Here's how the part is built. I have some questions about the finished solid (model axes, mm). Coordinates: 2 decimals unless noted, no trailing zeros. Write each loop counter-clockwise with the first axis right and the second up, starting at its lowest first coordinate (ties: lowest second). Pieces come first, ordered by that corner, then holes. Notation, with made-up numbers: M 5,-10 L 62,-10 A28 cw 62,10 Z; hole C 34,30 d6. An arc over 180 degrees is marked long. Use one line per item in the form item = value. Start each with the question number.
1. I want a section at C-C, the plane x = 12. List the corners of the cut face in (y, z) for me, plus the area to 3 significant figures.
2. Please list where these lines run through material, in increasing order: line 1 along X through (y, z) = (0.3, 8); line 2 along X through (y, z) = (0.7, -5); line 3 along Z through (x, y) = (27, 0.65). Write a range as [from, to].
3. I want a section at A-A, the plane z = -3.5. List the corners of the cut face in (x, y) for me.
4. I want a section at B-B, the plane y = 0.2. List the corners of the cut face in (x, z) for me, plus the area to 3 significant figures.
from build123d import *

# Parameters (mm, degrees)
SKETCH1_W            = 240
SKETCH1_H            = 65
BOSS_EXTRUDE1_DEPTH  = 1
M4_CLEARANCE_SLOT1_D = 4.8
SKETCH4_R            = 17.5
CUT_EXTRUDE1_DEPTH   = 5


with BuildPart() as part:
    # Sketch1 → Boss-Extrude1 (new body)
    with BuildSketch(Plane(origin=(0, 0, 0), x_dir=(1, 0, 0), z_dir=(0, 1, 0))):
        with Locations((-52.116935484, -7.731854839)):
            Rectangle(SKETCH1_W, SKETCH1_H)
    extrude(amount=BOSS_EXTRUDE1_DEPTH)

    # M4 Clearance Slot1 (through all)
    with Locations(Plane(origin=(0, 1, 0), x_dir=(1, 0, 0), z_dir=(0, 1, 0))):
        with Locations((-160.116935484, 12.768145161), (55.883064516, -28.231854839)):
            Hole(M4_CLEARANCE_SLOT1_D / 2)

    # Sketch4 → Cut-Extrude1 (cut)
    with BuildSketch(Plane(origin=(0, 1, 0), x_dir=(1, 0, 0), z_dir=(0, 1, 0))):
        with Locations(Location((15.883064516, -7.731854839, 0), (0, 0, 270))):
            Circle(SKETCH4_R)
    extrude(amount=-CUT_EXTRUDE1_DEPTH, mode=Mode.SUBTRACT)


solid = part.part
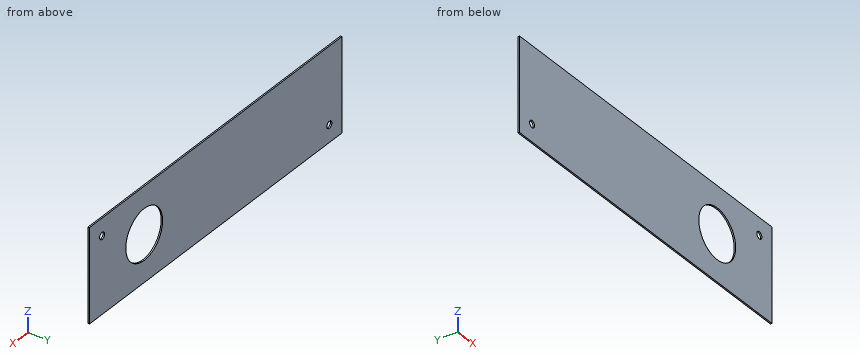
Answer list:
q1.outline = M 0,-24.77 L 1,-24.77 L 1,-9.33 L 0,-9.33 Z; M 0,24.8 L 1,24.8 L 1,40.23 L 0,40.23 Z
q1.area = 30.9 mm²
q2.line_1 = [-172.12, -1.61], [33.38, 67.88]
q2.line_2 = [-172.12, 3.88], [27.89, 67.88]
q2.line_3 = [-24.77, -5.78], [21.25, 40.23]
q3.outline = M -172.12,0 L 2.46,0 L 2.46,1 L -172.12,1 Z; M 29.3,0 L 67.88,0 L 67.88,1 L 29.3,1 Z
q4.outline = M -172.12,-24.77 L 67.88,-24.77 L 67.88,40.23 L -172.12,40.23 Z; hole C -160.12,-12.77 d4.8; hole C 15.88,7.73 d35; hole C 55.88,28.23 d4.8
q4.area = 14,600 mm²
